from build123d import *

# Parameters (mm, degrees)
BOSS_EXTRU_1_DEPTH      = 5
ESQUISSE2_R             = 1.5
ENL_V_MAT_EXTRU_1_DEPTH = 10


with BuildPart() as part:
    # Esquisse1 → Boss.-Extru.1 (new body)
    with BuildSketch(Plane(origin=(0, 0, 0), x_dir=(1, 0, 0), z_dir=(0, 1, 0))):
        Polygon((-124.568322948, 150), (-124.568322948, 130), (-144.568322948, 130), (-144.568322948, 40), (-104.568322948, 40), (-104.568322948, -40), (-144.568322948, -40), (-144.568322948, -130), (-124.568322948, -130), (-124.568322948, -150), (124.568322948, -150), (124.568322948, -130), (144.568322948, -130), (144.568322948, -40), (104.568322948, -40), (104.568322948, 40), (144.568322948, 40), (144.568322948, 130), (124.568322948, 130), (124.568322948, 150), align=None)
    extrude(amount=BOSS_EXTRU_1_DEPTH)

    # Esquisse2 → Enlèv. mat.-Extru.1 (cut)
    with BuildSketch(Plane(origin=(0, 5, 0), x_dir=(1, 0, 0), z_dir=(0, 1, 0))):
        with Locations(Location((-93.068322948, 8.042853971, 0), (0, 0, 270))):
            Circle(ESQUISSE2_R)
        with Locations(Location((-93.068322948, -8.042853971, 0), (0, 0, 270))):
            Circle(ESQUISSE2_R)
        with Locations(Location((-79.568322948, -8.042853971, 0), (0, 0, 270))):
            Circle(ESQUISSE2_R)
        with Locations(Location((-79.568322948, 8.042853971, 0), (0, 0, 270))):
            Circle(ESQUISSE2_R)
        with Locations(Location((93.068322948, -8.042853971, 0), (0, 0, 270))):
            Circle(ESQUISSE2_R)
        with Locations(Location((79.568322948, -8.042853971, 0), (0, 0, 270))):
            Circle(ESQUISSE2_R)
        with Locations(Location((79.568322948, 8.042853971, 0), (0, 0, 270))):
            Circle(ESQUISSE2_R)
        with Locations(Location((93.068322948, 8.042853971, 0), (0, 0, 270))):
            Circle(ESQUISSE2_R)
        with BuildLine():
            ThreePointArc((7.970010145, -128.811194391), (7.021605285, -128.408236457), (6.3113263, -127.661677259))
            ThreePointArc((6.3113263, -127.661677259), (0.055762197, -124.184876889), (-6.199801905, -127.661677259))
            ThreePointArc((-6.199801905, -127.661677259), (-6.910080891, -128.408236457), (-7.85848575, -128.811194391))
            ThreePointArc((-7.85848575, -128.811194391), (-10.104237803, -131.550876889), (-7.85848575, -134.290559386))
            ThreePointArc((-7.85848575, -134.290559386), (-6.910080891, -134.69351732), (-6.199801905, -135.440076518))
            ThreePointArc((-6.199801905, -135.440076518), (0.055762197, -138.916876889), (6.3113263, -135.440076518))
            ThreePointArc((6.3113263, -135.440076518), (7.021605285, -134.69351732), (7.970010145, -134.290559386))
            ThreePointArc((7.970010145, -134.290559386), (10.215762197, -131.550876889), (7.970010145, -128.811194391))
        make_face()
        with BuildLine():
            ThreePointArc((7.970010145, 128.811194391), (10.215762197, 131.550876889), (7.970010145, 134.290559386))
            ThreePointArc((7.970010145, 134.290559386), (7.021605285, 134.69351732), (6.3113263, 135.440076518))
            ThreePointArc((6.3113263, 135.440076518), (0.055762197, 138.916876889), (-6.199801905, 135.440076518))
            ThreePointArc((-6.199801905, 135.440076518), (-6.910080891, 134.69351732), (-7.85848575, 134.290559386))
            ThreePointArc((-7.85848575, 134.290559386), (-10.104237803, 131.550876889), (-7.85848575, 128.811194391))
            ThreePointArc((-7.85848575, 128.811194391), (-6.910080891, 128.408236457), (-6.199801905, 127.661677259))
            ThreePointArc((-6.199801905, 127.661677259), (0.055762197, 124.184876889), (6.3113263, 127.661677259))
            ThreePointArc((6.3113263, 127.661677259), (7.021605285, 128.408236457), (7.970010145, 128.811194391))
        make_face()
    extrude(amount=-ENL_V_MAT_EXTRU_1_DEPTH, mode=Mode.SUBTRACT)


solid = part.part
Design review of the part built by this model. Coordinates are the model's own, in mm. Coordinates: 2 decimals unless noted, no trailing zeros. Write each loop counter-clockwise with the first axis right and the second up, starting at its lowest first coordinate (ties: lowest second). Pieces come first, ordered by that corner, then holes. Notation, with made-up numbers: (3.25, 6) - (34.25, 6) arc R11 cw to (34.25, 18) - close; hole circle Ø7 at (-34, -27). An arc over 180 degrees is marked (long way). One line per item, written item: value.
1) Add section A-A (z = 19). State the section outline as (x, y) points, plus the area to 3 significant figures.
Answer sheet:
outline: (-104.57, 0) - (104.57, 0) - (104.57, 5) - (-104.57, 5) - close
area: 1,050 mm2
2) Add section B-B (y = 1.6). Give the number of separate pieces and of enclosed holes in the cut face, plus the area to 3 significant figures.
Answer sheet:
separate pieces: 1
enclosed holes: 10
area: 78,300 mm2
3) Insertion check: pin 1 (1.5 mm diameter, centred on y = 2, z = -8, fed in from +X); pin 2 (3.5 mm diameter, centred on x = 79.57, z = 8.04, fed in from -Y); pin 3 (2.5 mm diameter, centred on x = 139, y = 3, fed in from +Z); pin 4 (1.5 mm diameter, centred on y = 1.5, z = -143, fed in from +X). Each pin has a flat end and moves straight along its axis. Give the tip position at first contact, or say it passes through.
Answer sheet:
pin 1: stops at x = 104.57
pin 2: stops at y = 0
pin 3: stops at z = 130
pin 4: stops at x = 124.57
4) To check wall thickness, follow probe 1 along Z at (x, y) = (-129, 4.1); probe 2 along Z at (x, y) = (7.5, 3.1); probe 3 along X at (y, z) = (3.5, -132). State the ranges of each line that lie inside material, in increasing order.
Answer sheet:
probe 1: z = -130 to -40, 40 to 130
probe 2: z = -150 to -134.43, -128.67 to 128.67, 134.43 to 150
probe 3: x = -124.57 to -10.07, 10.18 to 124.57
